from build123d import *

# Parameters (mm, degrees)
F0_W     = 101.6
F0_H     = 76.2
F1_DEPTH = 6.35
F3_DEPTH = 25.4
F5_DEPTH = 25.4


with BuildPart() as f1:
    # F0 (on Right) → F1 (new body)
    with BuildSketch(Plane.YZ):
        Rectangle(F0_W, F0_H)
    extrude(amount=F1_DEPTH)

    # F2 (on face) → F3 (cut)
    with BuildSketch(Plane.YZ.offset(6.35)):
        with BuildLine():
            Line((42.798216, 3.81), (-42.798216, 3.81))
            ThreePointArc((-42.798216, 3.81), (-46.608216, 0), (-42.798216, -3.81))
            Line((-42.798216, -3.81), (42.798216, -3.81))
            ThreePointArc((42.798216, -3.81), (46.608216, 0), (42.798216, 3.81))
        make_face()
    extrude(amount=-F3_DEPTH, mode=Mode.SUBTRACT)

    # F4 (on face) → F5 (cut)
    with BuildSketch(Plane.YZ.offset(6.35)):
        with BuildLine():
            Line((-42.798216, 5.068473), (42.798216, 5.068473))
            ThreePointArc((42.798216, 5.068473), (43.433216, 5.703473), (42.798216, 6.338473))
            Line((42.798216, 6.338473), (-42.798216, 6.338473))
            ThreePointArc((-42.798216, 6.338473), (-43.433216, 5.703473), (-42.798216, 5.068473))
        make_face()
    extrude(amount=-F5_DEPTH, mode=Mode.SUBTRACT)


solid = f1.part
Design review of the part built by this model. Coordinates are the model's own, in mm. A direction names the side the tool comes from. Round coordinates to 2 decimals unless told otherwise and drop trailing zeros. Loops run counter-clockwise (first coordinate to the right, second up) from the corner with the lowest first, then second, coordinate; pieces in that order, holes last. Notation, with made-up numbers: (39, 2.25) - (46, 2.25) arc R16 ccw to (46, 11.25) - close; hole circle Ø1 at (16, 22). An arc over 180 degrees is marked (long way). One line per item, written item: value. Start each with the question number.
1) To check wall thickness, follow L1, parallel to Z at x = 1.75, y = -32; L2, parallel to Y at x = 0.75, z = -3.5; L3, parallel to Y at x = 5.5, z = 1.5. State the ranges of each line that lie inside material, in increasing order. Write a range as from..to.
2) For faces 5 (the flat face through (3, -1, -38.1)), 6 (the flat face through (3, 1, 6.338)), list the 3-axis set-ups (+Z, -Z, +X, -X, +Y, -Y) from which the entire face can be reached by the end or side of a thin tool; tool diameter is ignored.
3) Consider section A-A on y = -27. Give the boundary of the cut face in (x, z), then the cut area to 3 significant figures.
4) Consider section B-B on x = 3. Give the boundary of the cut face in (y, z) (3 decimals).
5) Consider section C-C on z = 0. Give the boundary of the cut face in (x, y), then the cut area to 3 significant figures.
6) Draft analysis for pull direction Y (two halves, no side actions). For faces 1 (the flat face through (3, 50.8, -1)), 2 (the cylindrical face through (3.219, -46.607, 0.084)), 3 (the flat face through (0, -1, 9)), 4 (the flat face through (3, -50.8, -1)), state which applies: +Y half, -Y half, draft (parallel to the pull), parting line (faces both ways), or undercut.
Reported:
1. L1: z = -38.1..-3.81, 3.81..5.07, 6.34..38.1
1. L2: y = -50.8..-44.3, 44.3..50.8
1. L3: y = -50.8..-46.3, 46.3..50.8
2. face 5: -Z, +X, -X, +Y, -Y
2. face 6: +X, -X
3. outline: (0, -38.1) - (6.35, -38.1) - (6.35, -3.81) - (0, -3.81) - close; (0, 3.81) - (6.35, 3.81) - (6.35, 5.07) - (0, 5.07) - close; (0, 6.34) - (6.35, 6.34) - (6.35, 38.1) - (0, 38.1) - close
3. area: 427 mm^2
4. outline: (-50.8, -38.1) - (50.8, -38.1) - (50.8, 38.1) - (-50.8, 38.1) - close; hole (-42.798, -3.81) - (42.798, -3.81) arc R3.81 ccw to (42.798, 3.81) - (-42.798, 3.81) arc R3.81 ccw to start; hole (-42.798, 5.068) - (42.798, 5.068) arc R0.635 ccw to (42.798, 6.338) - (-42.798, 6.338) arc R0.635 ccw to start
5. outline: (0, -50.8) - (6.35, -50.8) - (6.35, -46.61) - (0, -46.61) - close; (0, 46.61) - (6.35, 46.61) - (6.35, 50.8) - (0, 50.8) - close
5. area: 53.2 mm^2
6. face 1: +Y half
6. face 2: undercut
6. face 3: draft
6. face 4: -Y half
